from build123d import *

# Parameters (mm, degrees)
BOX002_W     = 9.5
BOX002_H     = 8
BOX002_DEPTH = 3
SKETCH008_W  = 8.045495
SKETCH008_H  = 10.974572
SKETCH008_R  = 1.530969
PAD008_DEPTH = 5


with BuildPart() as body046:
    # Box002 → Box002 (new body)
    with BuildSketch(Plane.XY):
        with Locations((4.75, 4)):
            Rectangle(BOX002_W, BOX002_H)
    extrude(amount=BOX002_DEPTH)


with BuildPart() as body046_1:
    # Body046 placement: moved
    add(body046.part.moved(Location((-4, -3.9, 1))))


with BuildPart() as cut006:
    # Sketch008 → Pad008 (new body)
    with BuildSketch(Plane.XY):
        with Locations((1.022447, -0.012719)):
            Rectangle(SKETCH008_W, SKETCH008_H)
        Circle(SKETCH008_R, mode=Mode.SUBTRACT)
    extrude(amount=PAD008_DEPTH)

    # Cut006: cut Body046
    add(body046_1.part, mode=Mode.SUBTRACT)


with BuildPart() as cut006_1:
    # Cut006 placement: moved
    add(cut006.part.moved(Location((0, 0.025, 0))))


solid = cut006_1.part
Here's how the part is built. I have some questions about the finished solid (model axes, mm). A direction names the side the tool comes from. Give positions to 0.01 mm unless a question says otherwise; leave off trailing zeros. Order: outer loops, then holes, each group sorted by start corner. A loop starts at its lowest first (then second) coordinate and runs counter-clockwise, first axis right, second up. Notation, with made-up numbers: M 27.25,-22.5 L 65.25,-22.5 A19 ccw 65.25,7.5 Z; hole C 80,-36.75 d10. An arc over 180 degrees is marked long. Answer as a JSON object with one key per item and string values. Group by question number.
1) We'd pull the mould along X, two halves only. Please class faces 1 (the cylindrical face through (-1.21, -0.91, 0.49)), 2 (the flat face through (5.045, -0.1, 0.8)), 3 (the flat face through (1, 5.5, 2)), 4 (the cylindrical face through (-1.21, -0.91, 4.49)): pulls with the +X half, pulls with the -X half, needs draft (parallel to the pull), parting line crosses it, or undercut.
2) Suppose I cut it at D-D, the plane y = 0.5. Write out the boundary of the cut face in (x, z).
3) Suppose I cut it at C-C, the plane y = 3. Write out the boundary of the cut face in (x, z).
4) On a 3-axis mill with a long thin cutter (end or side, diameter ignored), from which of +Z, -Z, +X, -X, +Y, -Y can I reach the whole of each face in a straight line? I mean faces 5 (the flat face through (-3, -0.1, 0.8)), 6 (the flat face through (2, 0, 1)). Say none if no direction works.
5) Suppose I cut it at A-A, the plane x = 0. Write out the boundary of the cut face in (y, z) (3 decimals).
6) Please list where these lines run through material, in increasing order: L1, parallel to Z at x = 3.25, y = 1; L2, parallel to Y at x = 0, z = 0.3 (3 decimals); L3, parallel to Y at x = 4, z = 3.5 (3 decimals). Write a range as [from, to].
7) Suppose I cut it at B-B, the plane z = 2.2. Write out the boundary of the cut face in (x, y) (3 decimals), plus the area to 3 significant figures.
Results found:
{
 "1": {"face 1": "undercut", "face 2": "pulls with the +X half", "face 3": "needs draft", "face 4": "undercut"},
 "2": {"outline": "M -3,0 L -1.46,0 L -1.46,1 L -3,1 Z; M -3,4 L -1.46,4 L -1.46,5 L -3,5 Z; M 1.46,0 L 5.05,0 L 5.05,1 L 1.46,1 Z; M 1.46,4 L 5.05,4 L 5.05,5 L 1.46,5 Z"},
 "3": {"outline": "M -3,0 L 5.05,0 L 5.05,1 L -3,1 Z; M -3,4 L 5.05,4 L 5.05,5 L -3,5 Z"},
 "4": {"face 5": "+Z, -Z, -X, +Y, -Y", "face 6": "+X, -X"},
 "5": {"outline": "M -5.475,0 L -1.506,0 L -1.506,1 L -3.875,1 L -3.875,4 L -1.506,4 L -1.506,5 L -5.475,5 Z; M 1.556,0 L 5.5,0 L 5.5,5 L 1.556,5 L 1.556,4 L 4.125,4 L 4.125,1 L 1.556,1 Z"},
 "6": {"L1": "[0, 1], [4, 5]", "L2": "[-5.475, -1.506], [1.556, 5.5]", "L3": "[-5.475, -3.875], [4.125, 5.5]"},
 "7": {"outline": "M -3,-5.475 L 5.045,-5.475 L 5.045,-3.875 L -3,-3.875 Z; M -3,4.125 L 5.045,4.125 L 5.045,5.5 L -3,5.5 Z", "area": "23.9 mm²"}
}
